Input: part model. Units: mm. Frame: model coordinates. Round coordinates to 2 decimals unless told otherwise and drop trailing zeros. Write each loop counter-clockwise with the first axis right and the second up, starting at its lowest first coordinate (ties: lowest second). Pieces come first, ordered by that corner, then holes. Notation, with made-up numbers: (82, -6.75) - (126, -6.75) arc R32 cw to (126, 30.25) - close; hole circle Ø10 at (34.5, 74.5). An arc over 180 degrees is marked (long way). Use one line per item in the form item = value.
```python
from build123d import *

# Parameters (mm, degrees)
F2_T     = -1
F3_R     = 6.5
F4_DEPTH = 5


with BuildPart() as f1:
    # F0 (on Front) → F1 (revolve)
    with BuildSketch(Plane.XZ):
        Polygon((0, 27.239302), (0, 0), (0, -24.760698), (7, -24.760698), (7, 27.239302), align=None)
    revolve(axis=Axis((0, 0, 13.619651), (0, 0, 1)))

    # F2
    f2_openings = [f1.faces().sort_by_distance(p)[0] for p in [
        (0, 0, 27.239302),
    ]]
    offset(amount=F2_T, openings=f2_openings)

    # F3 (on face) → F4 (cut)
    with BuildSketch(Plane.XY.offset(27.239302)):
        Circle(F3_R)
    extrude(amount=-F4_DEPTH, mode=Mode.SUBTRACT)


solid = f1.part
```
(1) Material intervals for L1, parallel to Y at x = 0, z = 23.35; L2, parallel to Y at x = 0, z = 9; L3, parallel to X at y = -1.75, z = -6.5, sorted ascending.
Derived:
L1 = -7 to -6.5, 6.5 to 7
L2 = -7 to -6, 6 to 7
L3 = -6.78 to -5.74, 5.74 to 6.78
(2) Draft query along Y for faces 1 (the face through (6.466, -2.681, 1.603)), 2 (the face through (0, 0, -24.761)), 3 (the face through (-5.158, -3.955, 24.774)). Return one class per face: released by +Y, released by -Y, zero draft, split by the parting line, or undercut.
Derived:
face_1 = split by the parting line
face_2 = zero draft
face_3 = undercut
(3) Cut plane C-C on z = -13.5. Output: boundary loops of the cut face in (x, y), then the cut area to 3 significant figures.
Derived:
outline = circle Ø14 at (0, 0); hole circle Ø12 at (0, 0)
area = 40.8 mm^2
(4) Cut plane A-A on x = 0. Output: boundary loops of the cut face in (y, z), then the cut area to 3 significant figures.
Derived:
outline = (-7, -24.76) - (7, -24.76) - (7, 27.24) - (6.5, 27.24) - (6.5, 22.24) - (6, 22.24) - (6, -23.76) - (-6, -23.76) - (-6, 22.24) - (-6.5, 22.24) - (-6.5, 27.24) - (-7, 27.24) - close
area = 111 mm^2
(5) First-contact query: pin 1 Ø2 at (x, z) = (1.5, 6.5) entering from -Y; pin 2 Ø1 at (x, y) = (5, 2) entering from +Z; pin 3 Ø4 at (x, z) = (-5.5, 17) entering from -Y; pin 4 Ø6 at (x, y) = (-3.5, 4) entering from +Z. Flat tips, straight axial feed; report the tip coordinate or a pass-through.
Derived:
pin_1 = -6.98
pin_2 = -23.76
pin_3 = -6.06
pin_4 = 27.24
